The listing builds one solid part. Answer for the finished solid, in the listing's coordinates (mm). Round coordinates to 2 decimals unless told otherwise and drop trailing zeros. Write each loop counter-clockwise with the first axis right and the second up, starting at its lowest first coordinate (ties: lowest second). Pieces come first, ordered by that corner, then holes. Notation, with made-up numbers: M -38,9 L 2,9 A25 ccw 2,24 Z; hole C 28,4 d7. An arc over 180 degrees is marked long. Put each result on its own line as item: value. Start each with the question number.
```python
from build123d import *

# Parameters (mm, degrees)
F1_DEPTH = 3
F3_DEPTH = 25
F5_DEPTH = 25
F7_DEPTH = 25


# Not quite as in the source:
# - a feature names something its author has since deleted; it is built from what else it names


with BuildPart() as f1:
    # F0 (on Top) → F1 (new body)
    with BuildSketch(Plane.XY):
        Polygon((-5, 1855.804875493), (-30, 1855.804875493), (-30, -144.195124507), (-5, -144.195124507), (-5, -164.195124507), (0, -164.195124507), (0, -144.195124507), (30, -144.195124507), (30, -164.195124507), (35, -164.195124507), (35, -144.195124507), (95, -144.195124507), (95, 1855.804875493), (0, 1855.804875493), (0, 1875.804875493), (-5, 1875.804875493), align=None)
    extrude(amount=F1_DEPTH)

    # F2 (on face) → F3 (join)
    with BuildSketch(Plane.XZ.offset(144.195124507)):
        with BuildLine():
            Line((35, 3), (35.0980762114, 3))
            ThreePointArc((35.0980762114, 3), (29.5, 1.5), (35.0980762114, 0))
            Line((35.0980762114, 0), (35, 0))
            Line((35, 0), (35, 3))
        make_face()
        with BuildLine():
            ThreePointArc((35.0980762114, 0), (35.3977774789, 0.7235428647), (35.5, 1.5))
            ThreePointArc((35.5, 1.5), (35.3977774789, 2.2764571353), (35.0980762114, 3))
            Line((35.0980762114, 3), (35, 3))
            Line((35, 3), (35, 0))
            Line((35, 0), (35.0980762114, 0))
        make_face()
    extrude(amount=F3_DEPTH)

    # F4 (on face) → F5 (join)
    with BuildSketch(Plane(origin=(0, 1855.804875493, 0), x_dir=(-1, 0, 0), z_dir=(0, 1, 0))):
        with BuildLine():
            Line((0, 3), (-0.0980762114, 3))
            ThreePointArc((-0.0980762114, 3), (-0.5, 1.5), (-0.0980762114, 0))
            Line((-0.0980762114, 0), (0, 0))
            Line((0, 0), (0, 3))
        make_face()
        with BuildLine():
            ThreePointArc((-0.0980762114, 0), (3.2764571353, -1.3977774789), (5.5, 1.5))
            ThreePointArc((5.5, 1.5), (3.2764571353, 4.3977774789), (-0.0980762114, 3))
            Line((-0.0980762114, 3), (0, 3))
            Line((0, 3), (0, 0))
            Line((0, 0), (-0.0980762114, 0))
        make_face()
    extrude(amount=F5_DEPTH)

    # F6 (on face) → F7 (join)
    with BuildSketch(Plane.XZ.offset(144.195124507)):
        with BuildLine():
            ThreePointArc((0.0783741164, 0), (0.3926737069, 0.7383586703), (0.5, 1.5336188953))
            ThreePointArc((0.5, 1.5336188953), (0.4027223964, 2.2913805262), (0.1171982072, 3))
            Line((0.1171982072, 3), (0, 3))
            Line((0, 3), (0, 0))
            Line((0, 0), (0.0783741164, 0))
        make_face()
        with BuildLine():
            Line((0, 3), (0.1171982072, 3))
            ThreePointArc((0.1171982072, 3), (-5.4997488132, 1.5724397355), (0.0783741164, 0))
            Line((0.0783741164, 0), (0, 0))
            Line((0, 0), (0, 3))
        make_face()
    extrude(amount=F7_DEPTH)


solid = f1.part
```
Item 1: Flat-ended cylindrical pins translate along their axes: pin 1 (0.5 mm diameter, centred on x = 31.5, z = 4, fed in from +Y); pin 2 (2.5 mm diameter, centred on x = 18, z = 1, fed in from -Y); pin 3 (1 mm diameter, centred on x = 5.5, y = 1197, fed in from -Z). Find the tip coordinate at first contact, or state that the pin passes through.
Item 2: Section A-A (y = 1498) is taken. Give the vertices of the cut face in (x, z).
Item 3: Consider line 1 along Z through (x, y) = (43.5, 219.5); line 2 along Y through (x, z) = (40, 1). Determine where each line is inside the solid, lowest interval first. Write a range as [from, to].
Item 4: Section B-B (x = 53) is taken. Give the vertices of the cut face in (y, z), and give its area (3 significant figures).
Output values:
1. pin 1: stops at y = -144.2
1. pin 2: stops at y = -144.2
1. pin 3: stops at z = 0
2. outline: M -30,0 L 95,0 L 95,3 L -30,3 Z
3. line 1: z = [0, 3]
3. line 2: y = [-144.2, 1855.8]
4. outline: M -144.2,0 L 1855.8,0 L 1855.8,3 L -144.2,3 Z
4. area: 6,000 mm^2
